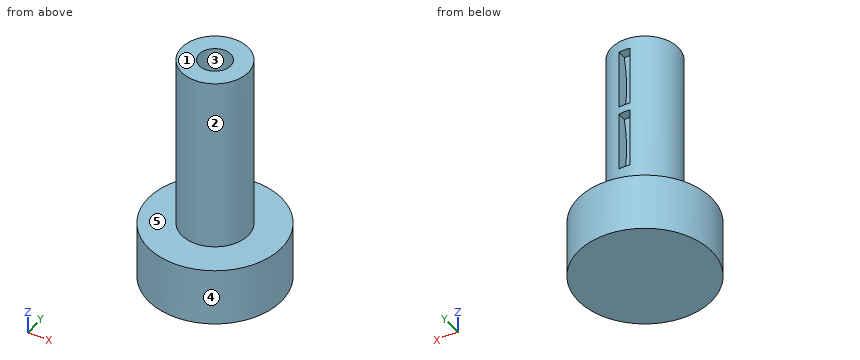
Autodesk Inventor part; units mm, degrees
ref_plane "YZ Plane" through (0, 0, 0) normal (1, 0, 0) x (0, 1, 0)
ref_plane "XZ Plane" through (0, 0, 0) normal (0, 1, 0) x (-1, 0, 0)
ref_plane "XY Plane" through (0, 0, 0) normal (0, 0, 1) x (1, 0, 0)
sketch "Эскиз1" plane through (0, 0, 0) normal (0, 0, 1) x (1, 0, 0)
  circle A0 centre (0, 0) radius 36
  dimension "d0" = 72
extrude "Выдавливание1" add sketch "Эскиз1" along normal blind 31
sketch "Эскиз2" plane through (0, 0, 31) normal (0, 0, 1) x (1, 0, 0)
  circle A0 centre (0, 0) radius 18
  dimension "d3" = 36
extrude "Выдавливание2" add sketch "Эскиз2" along normal blind 95
sketch "Эскиз3" plane through (0, 0, 126) normal (0, 0, 1) x (1, 0, 0)
  point P0 (0, -47.75)
  point P1 (0, 0)
hole "Отверстие1" at (0, 0, 126) direction (0, 0, -1) diameter 17 depth 31 tip angle 118
sketch "Эскиз4" plane through (0, 0, 0) normal (1, 0, 0) x (0, 1, 0)
  line L0 (18, 31) -> (18, 126)
  line L1 (18, 120) -> (18, 88)
  line L2 (18, 126) -> (-18, 126)
  line L3 (18, 120) -> (13, 120)
  line L4 (13, 120) -> (13, 88)
  line L5 (13, 88) -> (18, 88)
  arc A0 (13, 120) -> (13, 88) centre (81.1469, 104) ccw
  line L6 (18, 84) -> (18, 52)
  line L7 (18, 84) -> (13, 84)
  line L8 (13, 84) -> (13, 52)
  line L9 (13, 52) -> (18, 52)
  arc A1 (13, 84) -> (13, 52) centre (81.1469, 68) ccw
  point P0 (0, 0)
  point P1 (19, 127)
  dimension "d13" = 6
  dimension "d14" = 32
  dimension "d15" = 5
  dimension "d16" = 70
  dimension "d17" = 32
  dimension "d18" = 5
  dimension "d19" = 70
  dimension "d20" = 4
extrude "Выдавливание3" cut sketch "Эскиз4" against normal mid plane 6
properties part number "Носок" material "Сталь, высокопрочная, низколегированная"
The listing builds one solid part. Answer for the finished solid, in the listing's coordinates (mm). Face numbers are marked on the shaded views. A direction names the side the tool comes from. Coordinates: 2 decimals unless noted, no trailing zeros. Loops run counter-clockwise (first coordinate to the right, second up) from the corner with the lowest first, then second, coordinate; pieces in that order, holes last. Notation, with made-up numbers: M -31,56.25 L -18,56.25 A21 cw -18,83.25 Z; hole C -19,72 d2. An arc over 180 degrees is marked long. Answer as a JSON object with one key per item and string values. Group by question number.
Item 1: Determine the mould class of the marked faces 1, 2 and 3 for opening direction X: +X half, -X half, draft (parallel to the pull), parting line (faces both ways), or undercut.
Item 2: Section D-D (y = -28.5) is taken. Write down the section's boundary in (x, z).
Item 3: Consider L1, parallel to Y at x = 0, z = 105.5; L2, parallel to Y at x = 0, z = 109; L3, parallel to Z at x = 19, y = -9. Determine where each line is inside the solid, lowest interval first.
Item 4: Section C-C (z = 21.5) is taken. Write down the section's boundary in (x, y).
Item 5: Each of these flat-tipped pins is pushed along its axis until it touches: P1, Ø3.5, axis at y = 15, z = 63.5, coming from the +X side; P2, Ø1.5, axis at x = 1.5, y = 15.5, coming from the -Z side; P3, Ø3.5, axis at y = 15.5, z = 102.5, coming from the +X side; P4, Ø2, axis at y = 16, z = 98, coming from the -X side. Where does it stop, or does it pass through?
Item 6: Which of the six approach directions +Z, -Z, +X, -X, +Y, -Y give full straight-line access (tool end or side, diameter ignored) to the marked faces 4 and 5?
Item 7: Section A-A (y = -11) is taken. Write down the section's boundary in (x, z), and give its area (3 significant figures).
Solved:
{
 "1": {"face 1": "draft", "face 2": "parting line", "face 3": "undercut"},
 "2": {"outline": "M -21.99,0 L 21.99,0 L 21.99,31 L -21.99,31 Z"},
 "3": {"L1": "y = -18 to -8.5, 8.5 to 11.16", "L2": "y = -18 to -8.5, 8.5 to 11.33", "L3": "z = 0 to 31"},
 "4": {"outline": "C 0,0 d72"},
 "5": {"P1": "stops at x = 12.18", "P2": "stops at z = 0", "P3": "stops at x = 11.62", "P4": "stops at x = -9.95"},
 "6": {"face 4": "+Z, -Z", "face 5": "+Z"},
 "7": {"outline": "M -34.28,0 L 34.28,0 L 34.28,31 L 14.25,31 L 14.25,126 L -14.25,126 L -14.25,31 L -34.28,31 Z", "area": "4,830 mm2"}
}
